from build123d import *

# Parameters (mm, degrees)
SKETCH5_R           = 3.302
SKETCH5_R_2         = 0.889
BOSS_EXTRUDE1_DEPTH = 1.5875


with BuildPart() as part:
    # Sketch5 → Boss-Extrude1 (new body)
    with BuildSketch(Plane(origin=(0, 0, 0), x_dir=(1, 0, 0), z_dir=(0, 1, 0))):
        with BuildLine():
            Line((101.6, 4.75), (-101.6, 4.75))
            ThreePointArc((-101.6, 4.75), (-107.95, -1.6), (-101.6, -7.95))
            Line((-101.6, -7.95), (-25, -7.95))
            ThreePointArc((-25, -7.95), (-20.249761899, -5.569494064), (-15, -4.75))
            Line((-15, -4.75), (15, -4.75))
            ThreePointArc((15, -4.75), (20.249761899, -5.569494064), (25, -7.95))
            Line((25, -7.95), (101.6, -7.95))
            ThreePointArc((101.6, -7.95), (107.95, -1.6), (101.6, 4.75))
        make_face()
        with Locations(Location((-101.6, -1.6, 0), (0, 0, 270))):
            Circle(SKETCH5_R, mode=Mode.SUBTRACT)
        with Locations(Location((0, 2.75, 0), (0, 0, 270))):
            Circle(SKETCH5_R_2, mode=Mode.SUBTRACT)
        with Locations(Location((101.6, -1.6, 0), (0, 0, 270))):
            Circle(SKETCH5_R, mode=Mode.SUBTRACT)
        with Locations(Location((0, -2.75, 0), (0, 0, 270))):
            Circle(SKETCH5_R_2, mode=Mode.SUBTRACT)
        with Locations(Location((-76.2, -1.6, 0), (0, 0, 270))):
            Circle(SKETCH5_R, mode=Mode.SUBTRACT)
        with Locations(Location((76.2, -1.6, 0), (0, 0, 270))):
            Circle(SKETCH5_R, mode=Mode.SUBTRACT)
    extrude(amount=BOSS_EXTRUDE1_DEPTH)


solid = part.part
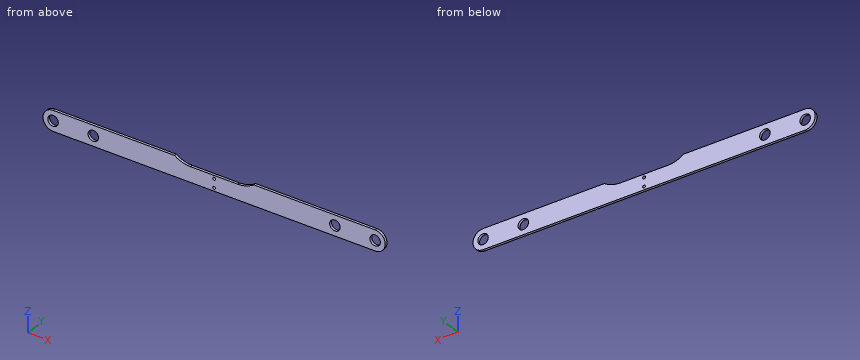
The listing builds one solid part. Answer for the finished solid, in the listing's coordinates (mm). Give positions to 0.01 mm unless a question says otherwise; leave off trailing zeros. Write each loop counter-clockwise with the first axis right and the second up, starting at its lowest first coordinate (ties: lowest second). Pieces come first, ordered by that corner, then holes. Notation, with made-up numbers: (-28, 78.25) -> (31, 78.25) arc R23 ccw to (31, 89.25) -> close; hole circle Ø8 at (3.5, 17). An arc over 180 degrees is marked (long way). Use a Markdown table: item, result.
(1) Section B-B, the plane x = 76.2 is taken. Determine the outline of the cut face in (y, z), then the cut area to 3 significant figures.
Return value:
| item | result |
|---|---|
| outline | (0, -4.75) -> (1.59, -4.75) -> (1.59, -1.7) -> (0, -1.7) -> close; (0, 4.9) -> (1.59, 4.9) -> (1.59, 7.95) -> (0, 7.95) -> close |
| area | 9.68 mm2 |
(2) Section C-C, the plane x = -8 is taken. Determine the outline of the cut face in (y, z), then the cut area to 3 significant figures.
Return value:
| item | result |
|---|---|
| outline | (0, -4.75) -> (1.59, -4.75) -> (1.59, 4.75) -> (0, 4.75) -> close |
| area | 15.1 mm2 |
(3) Find the intervals of material crossed by probe 1 along X at (y, z) = (0.5, 1.6); probe 2 along X at (y, z) = (0.75, 3.75); probe 3 along X at (y, z) = (1.1, 2.25), in increasing order. Write a range as from..to.
Return value:
| item | result |
|---|---|
| probe 1 | -107.95..-104.9, -98.3..-79.5, -72.9..72.9, 79.5..98.3, 104.9..107.95 |
| probe 2 | -107.57..-104.11, -99.09..-78.71, -73.69..73.69, 78.71..99.09, 104.11..107.57 |
| probe 3 | -107.92..-104.84, -98.36..-79.44, -72.96..-0.74, 0.74..72.96, 79.44..98.36, 104.84..107.92 |
(4) Section A-A, the plane y = 0.25 is taken. Determine the outline of the cut face in (x, z) (3 decimals), then the cut area to 3 significant figures.
Return value:
| item | result |
|---|---|
| outline | (-101.6, -4.75) -> (101.6, -4.75) arc R6.35 ccw to (101.6, 7.95) -> (25, 7.95) arc R17.225 cw to (15, 4.75) -> (-15, 4.75) arc R17.225 cw to (-25, 7.95) -> (-101.6, 7.95) arc R6.35 ccw to start; hole circle Ø6.604 at (-101.6, 1.6); hole circle Ø6.604 at (-76.2, 1.6); hole circle Ø1.778 at (0, -2.75); hole circle Ø1.778 at (0, 2.75); hole circle Ø6.604 at (76.2, 1.6); hole circle Ø6.604 at (101.6, 1.6) |
| area | 2,430 mm2 |
